Part model, mm, in its own coordinate system. A direction names the side the tool comes from. Round coordinates to 2 decimals unless told otherwise and drop trailing zeros. Loops run counter-clockwise (first coordinate to the right, second up) from the corner with the lowest first, then second, coordinate; pieces in that order, holes last. Notation, with made-up numbers: M 85.5,-25 L 117.5,-25 A3 ccw 117.5,-21 Z; hole C 68,62.5 d5. An arc over 180 degrees is marked long. Answer as CSV lines item,"result". Start each with the question number.
Item 1: Wall check: line 1 (Y direction, x = 5.5, z = 8.25); line 2 (X direction, y = 2.5, z = 7); line 3 (Z direction, x = 1, y = -11). Give the ranges that are in metal, low to high.
Item 2: Band-saw the part on B-B (y = -6). Give the cut face in (x, z), and give its area (3 significant figures).
Item 3: Which spindle directions (+Z, -Z, +X, -X, +Y, -Y) get a long thin tool onto all of the face, cutting with end or side? Do faces 1 (the flat face through (0, 4, 11)), 2 (the flat face through (3, 0, -7)). Say none if no direction does.
Item 4: Drop flat-ended pins along their axis: pin 1 Ø3 at (y, z) = (-4, -1.5) entering from +X; pin 2 Ø6 at (y, z) = (4.5, 8.5) entering from -X; pin 3 Ø5 at (y, z) = (-17.5, -8.5) entering from +X. Give the stop position or say it passes through.
Item 5: Band-saw the part on A-A (x = 0). Give the cut face in (y, z), and give its area (3 significant figures).
```python
from build123d import *

# Parameters (mm, degrees)
EXTRUDE_1_DEPTH = 9.09
SKETCH_2_R      = 7
EXTRUDE_2_DEPTH = 25
CHAMFER_1_SIZE  = 0.2
FILLET_1_R      = 0.2


with BuildPart() as part:
    # 草图1 → 凸台-拉伸1 (new body)
    with BuildSketch(Plane(origin=(0, 0, 0), x_dir=(1, 0, 0), z_dir=(0, 1, 0))):
        Polygon((12.701705922, 0), (6.350852961, 11), (-6.350852961, 11), (-12.701705922, 0), (-6.350852961, -11), (6.350852961, -11), align=None)
    extrude(amount=EXTRUDE_1_DEPTH)

    # 草图2 → 凸台-拉伸2 (add)
    with BuildSketch(Plane.XZ):
        with Locations(Location((0, 0, 0), (0, 0, 270))):
            Circle(SKETCH_2_R)
    extrude(amount=EXTRUDE_2_DEPTH)

    # 倒角1
    chamfer_1_edges = [part.edges().sort_by_distance(p)[0] for p in [
        (0, 0, 7),
        (0, -25, 7),
    ]]
    chamfer(chamfer_1_edges, length=CHAMFER_1_SIZE)

    # 圆角1
    fillet_1_edges = [part.edges().sort_by_distance(p)[0] for p in [
        (0, 0, 7.2),
        (0, 0, 11),
        (-9.526279442, 0, 5.5),
        (-9.526279442, 0, -5.5),
        (0, 0, -11),
        (9.526279442, 0, -5.5),
        (9.526279442, 0, 5.5),
    ]]
    fillet(fillet_1_edges, radius=FILLET_1_R)

    # 草图3 → 切除-旋转1 (revolve, cut)
    with BuildSketch(Plane.XY, mode=Mode.PRIVATE) as cut_revolve_1_sk:
        Polygon((10.201705922, 9.09), (12.701705922, 9.09), (12.701705922, 8.09), align=None)
    revolve(cut_revolve_1_sk.sketch.rotate(Axis((0, 0, 0), (0, 1, 0)), 270), axis=Axis((0, 0, 0), (0, 1, 0)), mode=Mode.SUBTRACT)


solid = part.part
```
Answer block:
1,line 1,"y = 0 to 9.09"
1,line 2,"x = -8.66 to 8.66"
1,line 3,"z = -6.93 to 6.93"
2,outline,"C 0,0 d14"
2,area,"154 mm^2"
3,face 1,"+Z, +X, -X, +Y, -Y"
3,face 2,"-Y"
4,pin 1,"stops at x = 7"
4,pin 2,"stops at x = -9.53"
4,pin 3,"stops at x = 3.61"
5,outline,"M -25,-6.8 L -24.8,-7 L -0.2,-7 L -0.06,-7.14 A0.2 cw 0,-7.28 L 0,-10.8 A0.2 ccw 0.2,-11 L 8.77,-11 L 9.09,-10.2 L 9.09,10.2 L 8.77,11 L 0.2,11 A0.2 ccw 0,10.8 L 0,7.28 A0.2 cw -0.06,7.14 L -0.2,7 L -24.8,7 L -25,6.8 Z"
5,area,"550 mm^2"
